```python
from build123d import *

# Parameters (mm, degrees)
CROQUIS4_OUTSIDE_W    = 60.478
CROQUIS4_OUTSIDE_H    = 60.478
CORTAR_EXTRUIR6_DEPTH = 70
CROQUIS5_OUTSIDE_W    = 199.794
CROQUIS5_OUTSIDE_H    = 193.9
CROQUIS5_OUTSIDE_R    = 19.052558883
CORTAR_EXTRUIR7_DEPTH = 70
CORTAR_EXTRUIR7_TAPER = 45
CROQUIS6_R            = 9
CORTAR_EXTRUIR8_DEPTH = 15
CHAFL_N1_SIZE         = 2
REDONDEO1_R           = 1


with BuildPart() as part:
    # Croquis1 → Revolución1 (revolve)
    with BuildSketch(Plane.XY):
        Polygon((6.35, 31.379194031), (20, 31.379194031), (22, 29.379194031), (22, 14.379194031), (20, 12.379194031), (14, 12.379194031), (13.076641816, 12.379194031), (13.076641816, 9.706334079), (14, 9.020543495), (14, -3.620805969), (12, -5.620805969), (1.5875, -5.620805969), (1.5875, 12.379194031), (6.35, 12.379194031), align=None)
    revolve(axis=Axis((0, 51.930492424, 0), (0, -1, 0)))

    # Croquis4 outside → Cortar-Extruir6 (cut)
    with BuildSketch(Plane(origin=(0, 31.379194031, 0), x_dir=(1, 0, 0), z_dir=(0, 1, 0))):
        Rectangle(CROQUIS4_OUTSIDE_W, CROQUIS4_OUTSIDE_H)
        Polygon((22, 0), (11, 19.052558883), (-11, 19.052558883), (-22, 0), (-11, -19.052558883), (11, -19.052558883), align=None, mode=Mode.SUBTRACT)
    extrude(amount=-CORTAR_EXTRUIR6_DEPTH, mode=Mode.SUBTRACT)

    # Croquis5 outside → Cortar-Extruir7 (cut)
    with BuildSketch(Plane(origin=(0, 31.379194031, 0), x_dir=(1, 0, 0), z_dir=(0, 1, 0))):
        Rectangle(CROQUIS5_OUTSIDE_W, CROQUIS5_OUTSIDE_H)
        Circle(CROQUIS5_OUTSIDE_R, mode=Mode.SUBTRACT)
    extrude(amount=-CORTAR_EXTRUIR7_DEPTH, taper=CORTAR_EXTRUIR7_TAPER, mode=Mode.SUBTRACT)

    # Croquis6 → Cortar-Extruir8 (cut)
    with BuildSketch(Plane(origin=(0, 31.379194031, 0), x_dir=(1, 0, 0), z_dir=(0, 1, 0))):
        Circle(CROQUIS6_R)
    extrude(amount=-CORTAR_EXTRUIR8_DEPTH, mode=Mode.SUBTRACT)

    # Chaflán1
    chafl_n1_edges = [part.edges().sort_by_distance(p)[0] for p in [
        (-9, 31.379194031, 0),
    ]]
    chamfer(chafl_n1_edges, length=CHAFL_N1_SIZE)

    # Redondeo1
    redondeo1_edges = [part.edges().sort_by_distance(p)[0] for p in [
        (-6.35, 16.379194031, 0),
    ]]
    fillet(redondeo1_edges, radius=REDONDEO1_R)


solid = part.part
```
Part model, mm, in its own coordinate system. A direction names the side the tool comes from. Give positions to 0.01 mm unless a question says otherwise; leave off trailing zeros. Write each loop counter-clockwise with the first axis right and the second up, starting at its lowest first coordinate (ties: lowest second). Pieces come first, ordered by that corner, then holes. Notation, with made-up numbers: M -0.5,34 L 13.5,34 A23 ccw 13.5,71 Z; hole C -8,30.25 d8. An arc over 180 degrees is marked long. Use CSV: the item, a comma, the result in double quotes.
Item 1: Drill centre lines: probe 1 along Z at (x, y) = (0, 0); probe 2 along Z at (x, y) = (0, 19); probe 3 along Y at (x, z) = (-12, 14). Where is each one in solid material? Low to high.
Taken from the geometry:
probe 1,"z = -14 to -1.59, 1.59 to 14"
probe 2,"z = -19.05 to -9, 9 to 19.05"
probe 3,"y = 12.38 to 31.38"
Item 2: Pin check, flat tips, straight feed: P1, Ø4, axis at x = -1, z = 3, coming from the +Y side; P2, Ø4, axis at y = 0, z = 2.5, coming from the -X side; P3, Ø16.5, axis at x = 0, z = 0, coming from the -Y side; P4, Ø14.5, axis at x = -2.5, z = 2.5, coming from the +Y side. Stop position of each tip, or through.
Taken from the geometry:
P1,"stops at y = 12.38"
P2,"stops at x = -13.99"
P3,"stops at y = -5.62"
P4,"stops at y = 31.16"
Item 3: Which spindle directions (+Z, -Z, +X, -X, +Y, -Y) get a long thin tool onto all of the face, cutting with end or side? Do faces 1 (the face through (14, 12.379, 0)), 2 (the face through (-1.172, 22.97, -8.923)), 3 (the face through (10.32, 12.92, 17.76)). Say none if no direction does.
Taken from the geometry:
face 1,"none"
face 2,"+Y"
face 3,"+Z, +X, -Y"
Item 4: Slice it at A-A on y = 19. Write the cut outline in (x, z).
Taken from the geometry:
outline,"M -22,0 L -11,-19.05 L 11,-19.05 L 22,0 L 11,19.05 L -11,19.05 Z; hole C 0,0 d18"
Item 5: Pull direction X, two halves, no side cores. Call faces 4 (the face through (-3, 16.379, 7)), 5 (the face through (-9.843, 30.663, 17.145)), 6 (the face through (19.77, 30.66, -0.05)), 7 (the face through (-0.34, 3.51, -1.55)): +X half, -X half, draft (parallel to the pull), parting line (faces both ways), or undercut.
Taken from the geometry:
face 4,"undercut"
face 5,"-X half"
face 6,"+X half"
face 7,"undercut"
